Autodesk Inventor part; units mm, degrees
ref_plane "YZ Plane" through (0, 0, 0) normal (1, 0, 0) x (0, 1, 0)
ref_plane "XZ Plane" through (0, 0, 0) normal (0, 1, 0) x (-1, 0, 0)
ref_plane "XY Plane" through (0, 0, 0) normal (0, 0, 1) x (1, 0, 0)
sketch "Sketch1" plane through (0, 0, 0) normal (0, 1, 0) x (-1, 0, 0)
  line L0 (0, 0) -> (0, -6.3397)
  line L1 (0, -6.3397) -> (15, -15)
  line L2 (25, 0) -> (0, 0)
  line L3 (25, 0) -> (25, -15)
  line L4 (25, -15) -> (15, -15)
  dimension "d1" = 60
  dimension "d25" = 15
  dimension "d26" = 10
  dimension "d27" = 15
extrude "Extrusion1" add sketch "Sketch1" along normal blind 7
sketch "Sketch2" plane through (-15, 0, -15) normal (0.5, 0, -0.866) x (-0.866, 0, -0.5)
  line L0 (-17.3205, 0) -> (0, 0)
  line L1 (0, 0) -> (0, 7)
  line L2 (-17.3205, 7) -> (0, 7)
  line L3 (-17.3205, 0) -> (-17.3205, 7)
  circle A0 centre (-3.6603, 3.5) radius 1.45
  circle A1 centre (-13.6603, 3.5) radius 1.45
  point P0 (-20.4904, 0)
  dimension "d5" = 2.9
  dimension "d6" = 10
  dimension "d8" = 7
  dimension "d9" = 3.5
  dimension "d10" = 17.3205
  dimension "d11" = 3.6603
extrude "Extrusion2" cut sketch "Sketch2" against normal through all contours A0 | A1
sketch "Sketch6" plane through (0, 7, 0) normal (0, 1, 0) x (1, 0, 0)
  line L0 (0, 0) -> (0, 6.3397)
  line L1 (0, 6.3397) -> (-15, 15)
  line L2 (-15, 15) -> (-25, 15)
  line L3 (-25, 15) -> (-25, 0)
  line L4 (-25, 0) -> (0, 0)
  line L5 (0, 6.3397) -> (-15, 15)
  line L6 (-25, 0) -> (0, 0)
  line L7 (-20.5, 15) -> (-20.5, 0)
  dimension "d34" = 4.5
extrude "Extrusion5" add sketch "Sketch6" along normal blind 7 contours L4 L3 L2 L7
sketch "Sketch8" plane through (-20.5, 7, 0) normal (1, 0, 0) x (0, 0, -1)
  line L0 (15, 0) -> (0, 0)
  line L1 (15, 0) -> (15, 7)
  line L2 (0, 7) -> (15, 7)
  line L3 (0, 0) -> (0, 7)
  circle A0 centre (7.5, 3.5) radius 1.75
  point P0 (0, -7)
  point P1 (0, 3.5)
  point P2 (7.5, 0)
  dimension "d35" = 3.5
extrude "Extrusion7" cut sketch "Sketch8" against normal through all contours A0
equation "\"d9\" = 0.5 * d8"
equation "\"d11\" = -0.5 * d6 + 0.5 * d10"
properties part number "LEDBracket" material "ABS Plastic"
The listing builds one solid part. Answer for the finished solid, in the listing's coordinates (mm). A direction names the side the tool comes from. Coordinates: 2 decimals unless noted, no trailing zeros. Order: outer loops, then holes, each group sorted by start corner. A loop starts at its lowest first (then second) coordinate and runs counter-clockwise, first axis right, second up.
Q1. A cutting plane is placed at D-D, the plane z = -4.75. State how many separate pieces and enclosed holes the cut face has, and give its area (3 significant figures).
Q2. For a pull along Z with two mould halves and no side action, classify faces 1 (the face through (-17, 3.9, -7)), 2 (the face through (-21, 5, -15)), 3 (the face through (-15, 5, 0)), 4 (the face through (-20.5, 9.7, -9.3)) as pulls with the +Z half, pulls with the -Z half, needs draft (parallel to the pull), parting line crosses it, or undercut.
Q3. Consider line 1 (Y direction, x = -21.7, z = -7.5); line 2 (X direction, y = 4.75, z = -3.5); line 3 (Y direction, x = -18.5, z = -6.75). Determine where each line is inside the solid, lowest interval first.
Q4. A cutting plane is placed at A-A, the plane y = 10.5. Write down the section's boundary in (x, z).
Q5. A cutting plane is placed at B-B, the plane y = 4.5. Write down the section's boundary in (x, z), and give its area (3 significant figures).
Q6. Which of the six approach directions +Z, -Z, +X, -X, +Y, -Y give full straight-line access (tool end or side, diameter ignored) to faces 5 (the face through (-12, 7, -6)), 6 (the face through (-22.7, 12, -8.4))?
Q7. Given P1, Ø5, axis at y = 5.5, z = -13, coming from the +X side, flat-ended and moving along its own axis, determine where the tip first touches the part or whether it passes through.
Q8. A cutting plane is placed at C-C, the plane y = 6.5. Write down the section's boundary in (x, z), and give its area (3 significant figures).
Answers follow:
1. separate pieces: 1
1. enclosed holes: 2
1. area: 191 mm2
2. face 1: undercut
2. face 2: pulls with the -Z half
2. face 3: pulls with the +Z half
2. face 4: needs draft
3. line 1: y = 0 to 8.75, 12.25 to 14
3. line 2: x = -25 to -18.26, -16.56 to -6.71, -5.02 to 0
3. line 3: y = 0 to 7
4. outline: (-25, -15) - (-20.5, -15) - (-20.5, -9.25) - (-25, -9.25) - close; (-25, -5.75) - (-20.5, -5.75) - (-20.5, 0) - (-25, 0) - close
5. outline: (-25, -15) - (-15, -15) - (-12.74, -13.69) - (-20.65, 0) - (-25, 0) - close; (-18.22, 0) - (-10.92, -12.64) - (-4.08, -8.69) - (-9.1, 0) - close; (-6.67, 0) - (-2.26, -7.64) - (0, -6.34) - (0, 0) - close
5. area: 258 mm2
6. face 5: +Z, -Z, +X, +Y
6. face 6: +X, -X
7. P1: stops at x = -7.21
8. outline: (-25, -15) - (-15, -15) - (0, -6.34) - (0, 0) - (-25, 0) - close
8. area: 310 mm2
